from build123d import *

# Parameters (mm, degrees)
PAD016_DEPTH    = 140
THICKNESS003_T  = -1.5
POCKET018_DEPTH = 5


with BuildPart() as part:
    # Sketch035 → Pad016 (new body)
    with BuildSketch(Plane.XY):
        with BuildLine():
            Line((-60, 52), (-60, -52))
            ThreePointArc((-60, -52), (-57.6568542495, -57.6568542495), (-52, -60))
            Line((-52, -60), (52, -60))
            ThreePointArc((52, -60), (57.6568542495, -57.6568542495), (60, -52))
            Line((60, -52), (60, 52))
            ThreePointArc((60, 52), (57.6568542495, 57.6568542495), (52, 60))
            Line((52, 60), (-52, 60))
            ThreePointArc((-52, 60), (-57.6568542495, 57.6568542495), (-60, 52))
        make_face()
    extrude(amount=PAD016_DEPTH)

    # Thickness003
    thickness003_openings = [part.faces().sort_by_distance(p)[0] for p in [
        (0, 0, 0),
    ]]
    offset(amount=THICKNESS003_T, openings=thickness003_openings)

    # Sketch046 (on Face10 of Thickness003) → Pocket018 (cut)
    with BuildSketch(Plane(origin=(0, 0, 0), x_dir=(1, 0, 0), z_dir=(0, 0, -1))):
        with BuildLine():
            Line((-52, -59), (52, -59))
            ThreePointArc((52, -59), (56.9497474683, -56.9497474683), (59, -52))
            Line((59, -52), (59, 52))
            ThreePointArc((59, 52), (56.9497474683, 56.9497474683), (52, 59))
            Line((52, 59), (-52, 59))
            ThreePointArc((-52, 59), (-56.9497474683, 56.9497474683), (-59, 52))
            Line((-59, 52), (-59, -52))
            ThreePointArc((-59, -52), (-56.9497474683, -56.9497474683), (-52, -59))
        make_face()
    extrude(amount=-POCKET018_DEPTH, mode=Mode.SUBTRACT)


solid = part.part
Build history of the part. All positions in model axes, mm. A direction names the side the tool comes from. Round coordinates to 2 decimals unless told otherwise and drop trailing zeros. Write each loop counter-clockwise with the first axis right and the second up, starting at its lowest first coordinate (ties: lowest second). Pieces come first, ordered by that corner, then holes. Notation, with made-up numbers: M 2,-27 L 20,-27 A6 ccw 20,-23 Z; hole C -4,49.5 d1. An arc over 180 degrees is marked long. Answer as a JSON object with one key per item and string values. Group by question number.
(1) Cut at B-B (x = 31.5). Give the cut face in (y, z), and give its area (4 significant figures).
(2) Which spindle directions (+Z, -Z, +X, -X, +Y, -Y) get a long thin tool onto all of the face, cutting with end or side? Do faces 1 (the flat face through (-1, 1, 140)), 2 (the flat face through (-1, -58.5, 71)). Say none if no direction does.
(3) Mould opens along Y. For faces 3 (the cylindrical face through (57.719, 57.594, 69.02)), 4 (the flat face through (-59, -1, 2)), 5 (the cylindrical face through (57.594, -57.719, 69.02)) say: pulls with the +Y half, pulls with the -Y half, needs draft (parallel to the pull), parting line crosses it, or undercut.
(4) Drill centre lines: L1, parallel to X at y = 3, z = 60; L2, parallel to Z at x = 25.5, y = 2.5. Where is each one in solid material? Low to high.
(5) Flat gauge pin, fed straight in: pin 1 (1.5 mm diameter, centred on x = -4.5, y = 42, fed in from -Z). Where does the tip first touch, or does it go through?
(6) Cut at A-A (z = 120). Give the cut face in (x, y), and give its area (3 significant figures).
Responses:
{
 "1": {"outline": "M -60,0 L -59,0 L -59,5 L -58.5,5 L -58.5,138.5 L 58.5,138.5 L 58.5,5 L 59,5 L 59,0 L 60,0 L 60,140 L -60,140 Z", "area": "590.5 mm2"},
 "2": {"face 1": "+Z, +X, -X, +Y, -Y", "face 2": "-Z"},
 "3": {"face 3": "pulls with the +Y half", "face 4": "undercut", "face 5": "pulls with the -Y half"},
 "4": {"L1": "x = -60 to -58.5, 58.5 to 60", "L2": "z = 138.5 to 140"},
 "5": {"pin 1": "stops at z = 138.5"},
 "6": {"outline": "M -60,-52 A8 ccw -52,-60 L 52,-60 A8 ccw 60,-52 L 60,52 A8 ccw 52,60 L -52,60 A8 ccw -60,52 Z; hole M -58.5,-52 A6.5 ccw -52,-58.5 L 52,-58.5 A6.5 ccw 58.5,-52 L 58.5,52 A6.5 ccw 52,58.5 L -52,58.5 A6.5 ccw -58.5,52 Z", "area": "692 mm2"}
}
